For this review, take the finished solid that the model builds, in its own axes (mm). Give positions to 0.01 mm unless a question says otherwise; leave off trailing zeros. Write each loop counter-clockwise with the first axis right and the second up, starting at its lowest first coordinate (ties: lowest second). Pieces come first, ordered by that corner, then holes.
Q1. We need section A-A (x = -98). Write out the cut boundary in (y, z) (3 decimals).
Q2. We need section B-B (y = 203). Write out the cut boundary in (x, z) (3 decimals), then the cut area to 3 significant figures.
Q3. Insertion check: P1, Ø12, axis at x = -143.5, y = -163.5, coming from the -Z side; P2, Ø1.5, axis at y = 84, z = 1.5, coming from the +X side. Each pin has a flat end and moves straight along its axis. Give the tip position at first contact, or say it passes through.
Q4. We need section D-D (x = 1). Write out the cut boundary in (y, z) (3 decimals), then the cut area to 3 significant figures.
Q5. For line 1 (Y direction, x = 145, z = 0.5); line 2 (X direction, y = 186, z = 0.35); line 3 (X direction, y = 206, z = 2.1), list the stretches that pass through material, from the lowest coordinate up.
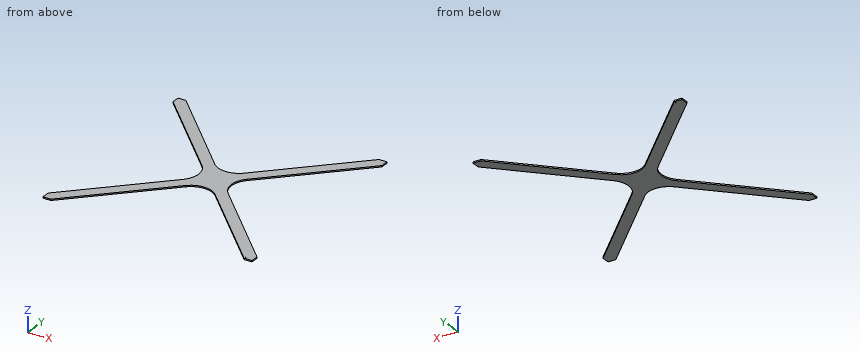
```python
from build123d import *

# Parameters (mm, degrees)
F0_W     = 508
F0_H     = 508
F1_DEPTH = 3.175
F3_DEPTH = 3.176
F4_R     = 50.8
F6_D     = 0.254


with BuildPart() as f1:
    # F0 (on Top) → F1 (new body)
    with BuildSketch(Plane.XY):
        Rectangle(F0_W, F0_H)
    extrude(amount=F1_DEPTH)

    # F2 (on face) → F3 (cut, through all)
    with BuildSketch(Plane.XY.offset(3.175)):
        Polygon((-19.05, 0), (-254, 234.95), (-254, -234.95), align=None)
        Polygon((-234.95, 254), (0, 19.05), (234.95, 254), align=None)
        Polygon((254, -234.95), (254, 234.95), (19.05, 0), align=None)
        Polygon((-234.95, -254), (234.95, -254), (0, -19.05), align=None)
    extrude(amount=-F3_DEPTH, mode=Mode.SUBTRACT)

    # F4
    f4_edges = [f1.edges().sort_by_distance(p)[0] for p in [
        (-19.05, 0, 1.5875),
        (0, -19.05, 1.5875),
        (19.05, 0, 1.5875),
        (0, 19.05, 1.5875),
    ]]
    fillet(f4_edges, radius=F4_R)

    # F6 (through all)
    with Locations(Plane(origin=(0, 0, 0), x_dir=(1, 0, 0), z_dir=(0, 0, -1))):
        with Locations((-247.698735, -244.907756), (-245.49396, -232.400599), (-233.360497, -236.151476), (-235.565272, -248.658633), (-245.49396, 248.658633), (-233.360497, 244.907756), (-235.565272, 232.400599), (-247.698735, 236.151476), (233.360497, -244.907756), (245.49396, -248.658633), (247.698735, -236.151476), (235.565272, -232.400599), (245.49396, 232.400599), (233.360497, 236.151476), (235.565272, 248.658633), (247.698735, 244.907756)):
            Hole(F6_D / 2)


solid = f1.part
```
Computed:
1. outline: (-117.05, 0) - (-78.95, 0) - (-78.95, 3.175) - (-117.05, 3.175) - close; (78.95, 0) - (117.05, 0) - (117.05, 3.175) - (78.95, 3.175) - close
2. outline: (-222.05, 0) - (-183.95, 0) - (-183.95, 3.175) - (-222.05, 3.175) - close; (183.95, 0) - (222.05, 0) - (222.05, 3.175) - (183.95, 3.175) - close
2. area: 242 mm2
3. P1: stops at z = 0
3. P2: stops at x = 103.8
4. outline: (-40.102, 0) - (40.102, 0) - (40.102, 3.175) - (-40.102, 3.175) - close
4. area: 255 mm2
5. line 1: y = -164.05 to -125.95, 125.95 to 164.05
5. line 2: x = -205.05 to -166.95, 166.95 to 205.05
5. line 3: x = -225.05 to -186.95, 186.95 to 225.05
